```python
from build123d import *

# Parameters (mm, degrees)
F0_W     = 75.692
F0_H     = 62.992
F1_DEPTH = 10.414
F3_DEPTH = 2.032
F4_R     = 19.05
F5_DEPTH = 15.24
F7_DEPTH = 50.292
F8_DEPTH = 34.544


with BuildPart() as f1:
    # F0 (on Front) → F1 (new body)
    with BuildSketch(Plane.XZ):
        with Locations((37.846, 31.496)):
            Rectangle(F0_W, F0_H)
    extrude(amount=F1_DEPTH)

    # F2 (on face) → F3 (join)
    with BuildSketch(Plane.XZ.offset(10.414)):
        with BuildLine():
            Line((49.784, 4.064), (70.612, 4.064))
            Line((70.612, 4.064), (70.612, 17.272))
            Line((70.612, 17.272), (62.339714, 17.272))
            ThreePointArc((62.339714, 17.272), (56.952336, 10.57447), (49.784, 5.831505))
            Line((49.784, 5.831505), (49.784, 4.064))
        make_face()
        with BuildLine():
            Line((5.08, 17.272), (5.08, 4.064))
            Line((5.08, 4.064), (25.908, 4.064))
            Line((25.908, 4.064), (25.908, 6.103985))
            ThreePointArc((25.908, 6.103985), (19.081744, 10.790558), (13.928818, 17.272))
            Line((13.928818, 17.272), (5.08, 17.272))
        make_face()
        with BuildLine():
            Line((25.908, 58.928), (5.08, 58.928))
            Line((5.08, 58.928), (5.08, 45.72))
            Line((5.08, 45.72), (14.247149, 45.72))
            ThreePointArc((14.247149, 45.72), (19.311604, 51.875193), (25.908, 56.349862))
            Line((25.908, 56.349862), (25.908, 58.928))
        make_face()
        with BuildLine():
            Line((70.612, 58.928), (49.784, 58.928))
            Line((49.784, 58.928), (49.784, 56.622342))
            ThreePointArc((49.784, 56.622342), (56.720072, 52.088644), (62.021382, 45.72))
            Line((62.021382, 45.72), (70.612, 45.72))
            Line((70.612, 45.72), (70.612, 58.928))
        make_face()
    extrude(amount=F3_DEPTH)

    # F4 (on face) → F5 (join)
    with BuildSketch(Plane.XZ.offset(10.414)):
        with Locations((38.134266, 31.226924)):
            Circle(F4_R)
    extrude(amount=F5_DEPTH)

    # F6 (on face) → F7 (join)
    with BuildSketch(Plane(origin=(0, 0, 0), x_dir=(-1, 0, 0), z_dir=(0, 1, 0))):
        with BuildLine():
            ThreePointArc((-42.164043, 37.927991), (-41.490457, 24.659777), (-30.099, 31.496))
            ThreePointArc((-30.099, 31.496), (-31.009777, 35.140457), (-33.527957, 37.927991))
            Line((-33.527957, 37.927991), (-42.164043, 37.927991))
        make_face()
    extrude(amount=F7_DEPTH)

    # F6 (on face) → F8 (join)
    with BuildSketch(Plane(origin=(0, 0, 0), x_dir=(-1, 0, 0), z_dir=(0, 1, 0))):
        with BuildLine():
            Line((-42.164043, 37.927991), (-33.527957, 37.927991))
            ThreePointArc((-33.527957, 37.927991), (-37.846, 39.243), (-42.164043, 37.927991))
        make_face()
    extrude(amount=F8_DEPTH)


solid = f1.part
```
Part model, mm, in its own coordinate system. A direction names the side the tool comes from. Coordinates: 2 decimals unless noted, no trailing zeros. Order: outer loops, then holes, each group sorted by start corner. A loop starts at its lowest first (then second) coordinate and runs counter-clockwise, first axis right, second up. Notation, with made-up numbers: (4.5, -5) -> (34.5, -5) arc R25 cw to (34.5, 22) -> close; hole circle Ø2 at (-13, 44). An arc over 180 degrees is marked (long way). Put each result on its own line as item: value. Start each with the question number.
(1) Band-saw the part on B-B (z = 55). Give the cut face in (x, y), then the cut area to 3 significant figures.
(2) Pin check, flat tips, straight feed: pin 1 Ø2 at (x, y) = (11, -11.5) entering from -Z; pin 2 Ø9.5 at (x, y) = (37.5, 44.5) entering from +Z; pin 3 Ø2 at (y, z) = (-11.5, 5) entering from +X. Stop position of each tip, or through.
(3) Probe line 1 along Y through (x, z) = (59, 32.5); line 2 along Y through (x, z) = (8, 56); line 3 along X through (y, z) = (40, 37). List the from-to ranges inside material, lowest first. Write a range as [from, to].
(4) Band-saw the part on C-C (y = 10). Give the cut face in (x, z), then the cut area to 3 significant figures.
(5) Band-saw the part on A-A (x = 10). Give the cut face in (y, z), then the cut area to 3 significant figures.
(6) Which spindle directions (+Z, -Z, +X, -X, +Y, -Y) get a long thin tool onto all of the face, cutting with end or side? Do faces 4 (the face through (13, -12.446, 54)), 5 (the face through (56.63, -11.42, 52.17)), 6 (the face through (70.612, -11, 52)), 7 (the face through (62, -12.446, 54)). Say none if no direction does.
(7) Band-saw the part on D-D (x = 37). Give the cut face in (y, z).
(8) Mould opens along X. For faces 1 (the face through (70.612, -11, 11)), 2 (the face through (10, -11, 45.72)), 3 (the face through (19.23, -11.42, 51.8)) say: pulls with the +X half, pulls with the -X half, needs draft (parallel to the pull), parting line crosses it, or undercut.
Determined:
1. outline: (0, -10.41) -> (5.08, -10.41) -> (5.08, -12.45) -> (23.45, -12.45) -> (23.45, -10.41) -> (52.81, -10.41) -> (52.81, -12.45) -> (70.61, -12.45) -> (70.61, -10.41) -> (75.69, -10.41) -> (75.69, 0) -> (0, 0) -> close
1. area: 862 mm²
2. pin 1: stops at z = 4.06
2. pin 2: stops at z = 37.93
2. pin 3: stops at x = 70.61
3. line 1: y = [-10.41, 0]
3. line 2: y = [-12.45, 0]
3. line 3: x = [32.39, 43.3]
4. outline: (30.1, 31.5) arc R7.75 ccw (long way) to (42.16, 37.93) arc R7.75 ccw to (33.53, 37.93) arc R7.75 ccw to start
4. area: 189 mm²
5. outline: (-12.45, 4.06) -> (-10.41, 4.06) -> (-10.41, 0) -> (0, 0) -> (0, 62.99) -> (-10.41, 62.99) -> (-10.41, 58.93) -> (-12.45, 58.93) -> (-12.45, 45.72) -> (-10.41, 45.72) -> (-10.41, 17.27) -> (-12.45, 17.27) -> close
5. area: 710 mm²
6. face 4: +Z, -X, -Y
6. face 5: -Y
6. face 6: +Z, -Z, +X, -Y
6. face 7: +Z, +X, -Y
7. outline: (-25.65, 12.21) -> (-10.41, 12.21) -> (-10.41, 0) -> (0, 0) -> (0, 23.8) -> (50.29, 23.8) -> (50.29, 37.93) -> (34.54, 37.93) -> (34.54, 39.2) -> (0, 39.2) -> (0, 62.99) -> (-10.41, 62.99) -> (-10.41, 50.24) -> (-25.65, 50.24) -> close
8. face 1: pulls with the +X half
8. face 2: needs draft
8. face 3: undercut
